Geometry: see drawing. Coordinates: mm, zero at the bounding-box minimum. A direction names the side the tool comes from. Round coordinates to 2 decimals unless told otherwise and drop trailing zeros. Loops run counter-clockwise (first coordinate to the right, second up) from the corner with the lowest first, then second, coordinate; pieces in that order, holes last. Notation, with made-up numbers: (64, 9.5) - (108, 9.5) arc R17 ccw to (108, 34.5) - close; hole circle Ø1 at (-17.75, 0.5). An arc over 180 degrees is marked (long way). Return JSON: item names as keys, results as strings. Group by question number.
1. Material intervals for probe 1 along Z at (x, y) = (12, 8); probe 2 along Z at (x, y) = (17.5, 31) (1 decimal); probe 3 along X at (y, z) = (7, 12), sorted ascending.
2. Section A-A on y = 3. Return loops of the section in (x, z), and give its area (3 significant figures).
3. First-contact query: pin 1 Ø8 at (x, y) = (4, 18) entering from +Z; pin 2 Ø4 at (x, y) = (13, 29.5) entering from -Z; pin 3 Ø2 at (x, y) = (11, 4) entering from -Z (1 decimal). Flat tips, straight axial feed; report the tip coordinate or a pass-through.
4. Section B-B on y = 13. Return loops of the section in (x, z), and give its area (3 significant figures).
5. Set-up query: the marked faces 1 and 2. Return all of +Z, -Z, +X, -X, +Y, -Y with unobstructed straight access to the full face (end or side cutting, diameter ignored); none if empty.
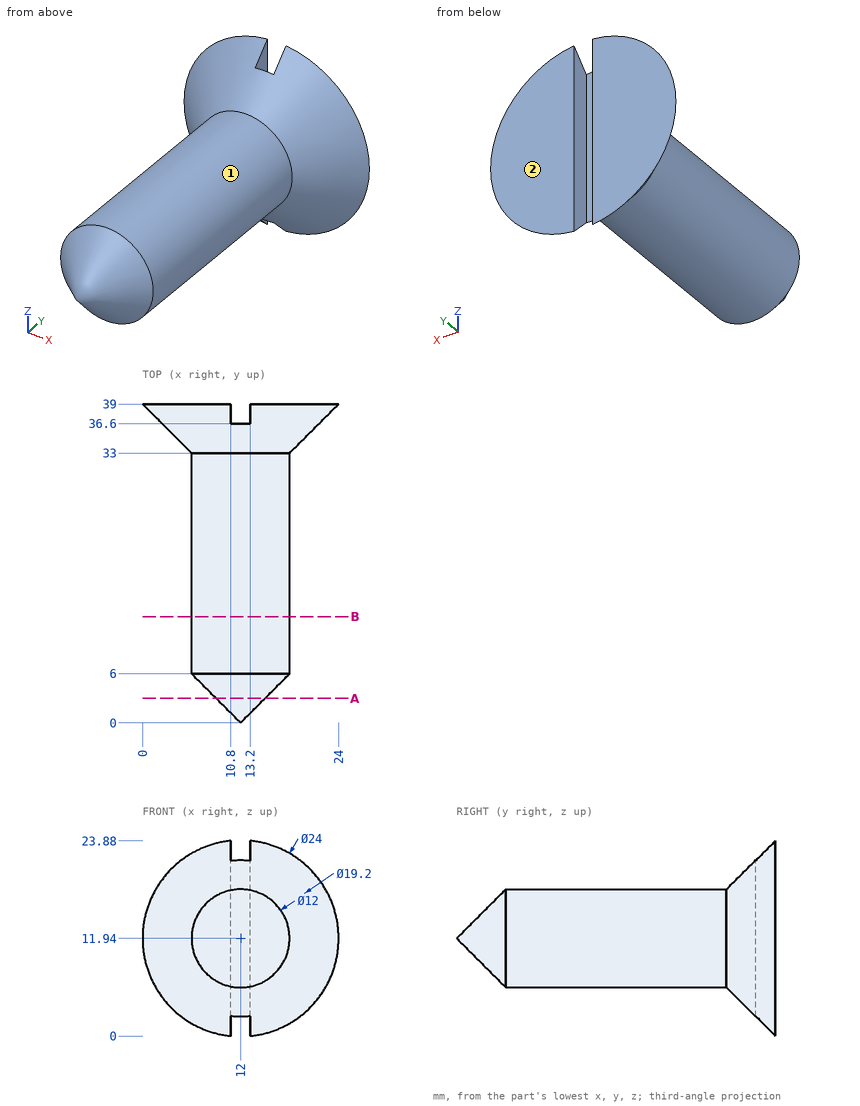
Taken from the geometry:
{
 "1": {"probe 1": "5.94 to 17.94", "probe 2": "9.5 to 14.3", "probe 3": "6 to 18"},
 "2": {"outline": "circle Ø6 at (12, 11.94)", "area": "28.3 mm2"},
 "3": {"pin 1": "z = 16.41", "pin 2": "z = 5.94", "pin 3": "z = 7"},
 "4": {"outline": "circle Ø12 at (12, 11.94)", "area": "113 mm2"},
 "5": {"face 1": "-Y", "face 2": "+Z, -Z, +X, -X, +Y"}
}
